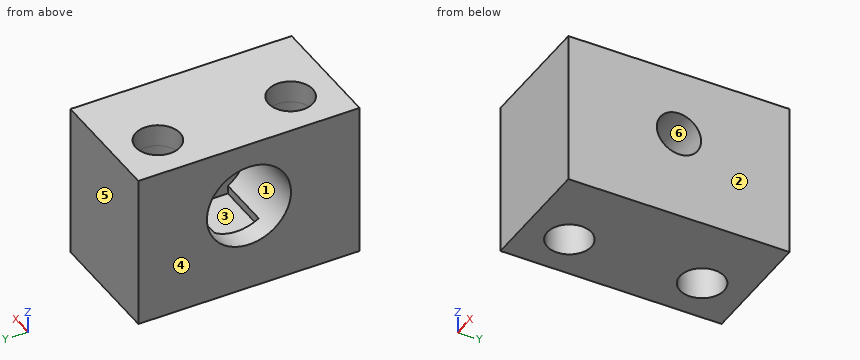
from build123d import *

# Parameters (mm, degrees)
MODEL_R                  = 1
EXTRUDE_1_DEPTH          = 4
SKETCH_1_R               = 1
CUT_EXTRUDE_1_DEPTH      = 5
CUT_EXTRUDE_1_DEPTH_BACK = 3
SKETCH_2_R               = 1.9
CUT_EXTRUDE_2_DEPTH      = 3.5
SKETCH_4_W               = 5.5
SKETCH_4_H               = 10
EXTRUDE_2_DEPTH          = 2
SKETCH_5_R               = 1
CUT_EXTRUDE_3_DEPTH      = 2
SKETCH_6_R               = 1
CUT_EXTRUDE_4_DEPTH      = 2
SKETCH_7_W               = 5.5
SKETCH_7_H               = 10
EXTRUDE_3_DEPTH          = 1
SKETCH_8_R               = 1
CUT_EXTRUDE_5_DEPTH      = 1


with BuildPart() as part:
    # Model → 凸台-拉伸1 (new body)
    with BuildSketch(Plane.XY):
        Polygon((199.499322294, 238.665580803), (199.499322294, 228.665580803), (193.999322294, 228.665580803), (193.999322294, 232.665580803), (193.999322294, 234.665580803), (193.999322294, 238.665580803), align=None)
        with Locations((195.999322294, 236.665580803)):
            Circle(MODEL_R, mode=Mode.SUBTRACT)
        with Locations((195.999322294, 230.665580803)):
            Circle(MODEL_R, mode=Mode.SUBTRACT)
        Polygon((195.999322294, 234.665580803), (197.499322294, 234.665580803), (197.499322294, 232.665580803), (195.999322294, 232.665580803), (194.999322294, 232.665580803), (194.999322294, 234.665580803), align=None, mode=Mode.SUBTRACT)
    extrude(amount=EXTRUDE_1_DEPTH)

    # 草图1 → 切除-拉伸1 (cut, two sides)
    with BuildSketch(Plane.ZY.offset(-197.499322294)) as cut_extrude_1_sk:
        with Locations((2, 233.665580803)):
            Circle(SKETCH_1_R)
    extrude(amount=CUT_EXTRUDE_1_DEPTH, mode=Mode.SUBTRACT)
    extrude(cut_extrude_1_sk.sketch, amount=-CUT_EXTRUDE_1_DEPTH_BACK, mode=Mode.SUBTRACT)

    # 草图2 → 切除-拉伸2 (cut)
    with BuildSketch(Plane.ZY.offset(-193.999322294)):
        with Locations((2, 233.665580803)):
            Circle(SKETCH_2_R)
    extrude(amount=-CUT_EXTRUDE_2_DEPTH, mode=Mode.SUBTRACT)

    # 草图4 → 凸台-拉伸2 (add)
    with BuildSketch(Plane(origin=(0, 0, 0), x_dir=(-1, 0, 0), z_dir=(0, 0, -1))):
        with Locations((-196.749322294, 233.665580803)):
            Rectangle(SKETCH_4_W, SKETCH_4_H)
    extrude(amount=EXTRUDE_2_DEPTH)

    # 草图5 → 切除-拉伸3 (cut)
    with BuildSketch(Plane.XY):
        with Locations((195.999322294, 236.665580803)):
            Circle(SKETCH_5_R)
    extrude(amount=-CUT_EXTRUDE_3_DEPTH, mode=Mode.SUBTRACT)

    # 草图6 → 切除-拉伸4 (cut)
    with BuildSketch(Plane.XY):
        with Locations((195.999322294, 230.665580803)):
            Circle(SKETCH_6_R)
    extrude(amount=-CUT_EXTRUDE_4_DEPTH, mode=Mode.SUBTRACT)

    # 草图7 → 凸台-拉伸3 (add)
    with BuildSketch(Plane.XY.offset(4)):
        with Locations((196.749322294, 233.665580803)):
            Rectangle(SKETCH_7_W, SKETCH_7_H)
    extrude(amount=EXTRUDE_3_DEPTH)

    # 草图8 → 切除-拉伸5 (cut)
    with BuildSketch(Plane(origin=(0, 0, 4), x_dir=(-1, 0, 0), z_dir=(0, 0, -1))):
        with Locations((-195.999322294, 236.665580803)):
            Circle(SKETCH_8_R)
        with Locations((-195.999322294, 230.665580803)):
            Circle(SKETCH_8_R)
    extrude(amount=-CUT_EXTRUDE_5_DEPTH, mode=Mode.SUBTRACT)


solid = part.part
Could you check a few things on this model? Use its own coordinates, in mm. Face numbers are marked on the shaded views. A direction names the side the tool comes from. Give positions to 0.01 mm unless a question says otherwise; leave off trailing zeros. Order: outer loops, then holes, each group sorted by start corner. A loop starts at its lowest first (then second) coordinate and runs counter-clockwise, first axis right, second up. Notation, with made-up numbers: (63, 30) - (69, 30) arc R22 cw to (69, 52) - close; hole circle Ø1 at (-34, 76). An arc over 180 degrees is marked (long way). Return JSON: item names as keys, results as strings. Group by question number.
Q1. Suppose I cut it at C-C, the plane y = 230.25. Please give me the cut outline in (x, z).
Q2. Which directions (+Z, -Z, +X, -X, +Y, -Y) give clear straight access to the entire face, cutting with the end or side of a thin tool? Please do the marked faces 1, 2 and 3.
Q3. Thinking about a two-plate mould opening in Y: for the marked faces 4, 5 and 6, which applies, pulls with the +Y half, pulls with the -Y half, needs draft (parallel to the pull), parting line crosses it, or undercut?
Q4. Suppose I cut it at A-A, the plane z = 2. Please give me the cut outline in (x, y), and give its area (3 significant figures).
Q5. Please list where these lines run through material, in increasing order: line 1 along Y through (x, z) = (195.25, 2.5); line 2 along X through (y, z) = (230.75, 1.75); line 3 along Y through (x, z) = (195.45, -0.75). Write a range as [from, to].
Q6. Will these pins go through, and if not, where does the flat tip stop? pin 1 Ø3 at (y, z) = (233.67, 2) entering from -X; pin 2 Ø1.8 at (x, y) = (196, 236.67) entering from +Z.
Q7. Suppose I cut it at D-D, the plane z = 0.75. Please give me the cut outline in (x, y).
Q8. Suppose I cut it at B-B, the plane x = 196.85. Please give me the cut outline in (y, z).
Resolved:
{
 "1": {"outline": "(194, -2) - (195.09, -2) - (195.09, 5) - (194, 5) - close; (196.91, -2) - (199.5, -2) - (199.5, 5) - (196.91, 5) - close"},
 "2": {"face 1": "-X", "face 2": "+Z, -Z, +X, +Y, -Y", "face 3": "none"},
 "3": {"face 4": "needs draft", "face 5": "pulls with the +Y half", "face 6": "undercut"},
 "4": {"outline": "(194, 228.67) - (199.5, 228.67) - (199.5, 232.67) - (197.5, 232.67) - (197.5, 231.77) - (194, 231.77) - close; (194, 235.57) - (197.5, 235.57) - (197.5, 234.67) - (199.5, 234.67) - (199.5, 238.67) - (194, 238.67) - close; hole circle Ø2 at (196, 230.67); hole circle Ø2 at (196, 236.67)", "area": "31.4 mm2"},
 "5": {"line 1": "y = [228.67, 230], [231.33, 231.83], [235.5, 236], [237.33, 238.67]", "line 2": "x = [194, 195], [197, 199.5]", "line 3": "y = [228.67, 229.83], [231.5, 235.83], [237.5, 238.67]"},
 "6": {"pin 1": "stops at x = 197.5", "pin 2": "passes through"},
 "7": {"outline": "(194, 228.67) - (199.5, 228.67) - (199.5, 238.67) - (194, 238.67) - (194, 235.1) - (197.5, 235.1) - (197.5, 232.23) - (194, 232.23) - close; hole circle Ø2 at (196, 230.67); hole circle Ø2 at (196, 236.67)"},
 "8": {"outline": "(228.67, -2) - (230.14, -2) - (230.14, 5) - (228.67, 5) - close; (231.19, -2) - (236.14, -2) - (236.14, 5) - (231.19, 5) - close; (237.19, -2) - (238.67, -2) - (238.67, 5) - (237.19, 5) - close; hole (232.67, 0) - (234.67, 0) - (234.67, 0.38) arc R1.9 ccw to (234.67, 3.62) - (234.67, 4) - (232.67, 4) - (232.67, 3.62) arc R1.9 ccw to (232.67, 0.38) - close"}
}
